from build123d import *

# Parameters (mm, degrees)
BOSS_EXTRUDE1_DEPTH = 6
SKETCH2_W           = 6
SKETCH2_H           = 40
CUT_EXTRUDE1_DEPTH  = 10


with BuildPart() as part:
    # Sketch1 → Boss-Extrude1 (new body)
    with BuildSketch(Plane.XY):
        Polygon((-350, 40), (-350, 14), (-337.96, 14), (-337.96, 40), (-281.96, 40), (-281.96, 14), (-269.92, 14), (-269.92, 40), (-179.92, 40), (-179.92, 14), (-167.88, 14), (-167.88, 40), (-80, 40), (-80, -40), (-380, -40), (-380, 40), align=None)
    extrude(amount=BOSS_EXTRUDE1_DEPTH)

    # Sketch2 → Cut-Extrude1 (cut)
    with BuildSketch(Plane(origin=(0, 0, 0), x_dir=(-1, 0, 0), z_dir=(0, 0, -1))):
        with Locations((57, 20)):
            Rectangle(SKETCH2_W, SKETCH2_H)
        with Locations((117, 20)):
            Rectangle(SKETCH2_W, SKETCH2_H)
    extrude(amount=-CUT_EXTRUDE1_DEPTH, mode=Mode.SUBTRACT)


solid = part.part
Build history of the part. All positions in model axes, mm. A direction names the side the tool comes from. Give positions to 0.01 mm unless a question says otherwise; leave off trailing zeros. Loops run counter-clockwise (first coordinate to the right, second up) from the corner with the lowest first, then second, coordinate; pieces in that order, holes last. Notation, with made-up numbers: (8, 0.5) - (41, 0.5) arc R16 ccw to (41, 23.5) - close; hole circle Ø10 at (60.5, -15). An arc over 180 degrees is marked (long way). Write item = value, one per line. Start each with the question number.
1) Probe probe 1 along X at (y, z) = (28, 4.7); probe 2 along X at (y, z) = (8, 2.05); probe 3 along Y at (x, z) = (-338, 4.7). List the from-to ranges inside material, lowest first. Write a range as from..to.
2) Band-saw the part on A-A on y = 21. Give the cut face in (x, z).
3) Band-saw the part on B-B on y = 4.5. Give the cut face in (x, z).
4) Tool access for faces 1 (the flat face through (-310, 40, 3)), 2 (the flat face through (-120, 20, 3)): list every direction of +Z, -Z, +X, -X, +Y, -Y with a clear straight run to the whole face (end or side of a thin tool).
5) Band-saw the part on C-C on z = 3.2. Give the cut face in (x, y), plus the area to 3 significant figures.
6) Drop a flat-ended pin along its axis: pin 1 Ø1.8 at (x, z) = (-274.5, 2) entering from +Y. Give the stop position or say it passes through.
7) Pull direction X, two halves, no side cores. Call faces 3 (the flat face through (-80, 1, 3)), 4 (the flat face through (-276, 14, 3)), 5 (the flat face through (-365, 40, 3)): +X half, -X half, draft (parallel to the pull), parting line (faces both ways), or undercut.
Final values:
q1.probe_1 = -380..-350, -337.96..-281.96, -269.92..-179.92, -167.88..-120, -114..-80
q1.probe_2 = -380..-120, -114..-80
q1.probe_3 = -40..14
q2.outline = (-380, 0) - (-350, 0) - (-350, 6) - (-380, 6) - close; (-337.96, 0) - (-281.96, 0) - (-281.96, 6) - (-337.96, 6) - close; (-269.92, 0) - (-179.92, 0) - (-179.92, 6) - (-269.92, 6) - close; (-167.88, 0) - (-120, 0) - (-120, 6) - (-167.88, 6) - close; (-114, 0) - (-80, 0) - (-80, 6) - (-114, 6) - close
q3.outline = (-380, 0) - (-120, 0) - (-120, 6) - (-380, 6) - close; (-114, 0) - (-80, 0) - (-80, 6) - (-114, 6) - close
q4.face_1 = +Z, -Z, +X, -X, +Y
q4.face_2 = +Z, -Z, +Y
q5.outline = (-380, -40) - (-80, -40) - (-80, 40) - (-114, 40) - (-114, 0) - (-120, 0) - (-120, 40) - (-167.88, 40) - (-167.88, 14) - (-179.92, 14) - (-179.92, 40) - (-269.92, 40) - (-269.92, 14) - (-281.96, 14) - (-281.96, 40) - (-337.96, 40) - (-337.96, 14) - (-350, 14) - (-350, 40) - (-380, 40) - close
q5.area = 22,800 mm²
q6.pin_1 = 14
q7.face_3 = +X half
q7.face_4 = undercut
q7.face_5 = draft
